Autodesk Inventor part; units mm, degrees
ref_plane "YZ Plane" through (0, 0, 0) normal (1, 0, 0) x (0, 1, 0)
ref_plane "XZ Plane" through (0, 0, 0) normal (0, 1, 0) x (-1, 0, 0)
ref_plane "XY Plane" through (0, 0, 0) normal (0, 0, 1) x (1, 0, 0)
sketch "Sketch1" plane through (0, 0, 0) normal (0, 1, 0) x (-1, 0, 0)
  circle A0 centre (0, 0) radius 6.35 construction
  line L0 (6.35, -3.6662) -> (0, -7.3323)
  line L1 (0, -7.3323) -> (-6.35, -3.6662)
  line L2 (-6.35, -3.6662) -> (-6.35, 3.6662)
  line L3 (-6.35, 3.6662) -> (0, 7.3323)
  line L4 (0, 7.3323) -> (6.35, 3.6662)
  line L5 (6.35, 3.6662) -> (6.35, -3.6662)
  circle A1 centre (0, 0) radius 9.525
  point P0 (6.35, 0)
  dimension "d0" = 12.7
  dimension "d1" = 19.05
extrude "Extrusion1" add sketch "Sketch1" along normal blind 9.525
properties part number "SportGearbox_HexDiffGearSpacer"
Geometry: final body of the model. Coordinates: model frame, mm. A direction names the side the tool comes from. Give positions to 0.01 mm unless a question says otherwise; leave off trailing zeros. Write each loop counter-clockwise with the first axis right and the second up, starting at its lowest first coordinate (ties: lowest second). Pieces come first, ordered by that corner, then holes.
1. Line query: probe 1 along X at (y, z) = (6.75, -2.25); probe 2 along X at (y, z) = (3.75, -0.25); probe 3 along Z at (x, y) = (1, 0.75). Output: solid intervals per line, ascending.
2. Section query B-B, the plane y = 5. Return loops of the section in (x, z) (3 decimals).
3. Section query A-A, the plane z = 0. Return loops of the section in (x, y) (3 decimals), then the cut area to 3 significant figures.
4. Section query C-C, the plane x = -3.5. Return loops of the section in (y, z) (3 decimals), then the cut area to 3 significant figures.
5. Pin query (flat end, axial travel): P1, Ø1, axis at x = -1.5, y = 8.5, coming from the -Z side; P2, Ø3, axis at y = 5.5, z = -4.5, coming from the +X side; P3, Ø2, axis at y = 7.5, z = 5.5, coming from the -X side (3 decimals). Return the tip coordinate at first contact, or that it passes through.
6. Draft query along Z for faces 3 (the flat face through (3.219, 4.696, 5.474)), 4 (the flat face through (6.35, 5, 0)), 5 (the cylindrical face through (7.559, 4.696, 5.796)), 6 (the flat face through (2.3, 0, -6.2)). Return one class per face: released by +Z, released by -Z, zero draft, split by the parting line, or undercut.
7. Reachability of faces 1 (the flat face through (-6.35, 5, 0)), 2 (the flat face through (2.3, 9.525, -6.2)) from +Z, -Z, +X, -X, +Y, -Y: full face, straight path, thin tool, end or side. Return the list, or none.
Computed:
1. probe 1: x = -9.26 to -6.35, 6.35 to 9.26
1. probe 2: x = -9.52 to -6.35, 6.35 to 9.52
1. probe 3: z = -9.47 to -6.75, 6.75 to 9.47
2. outline: circle Ø19.05 at (0, 0); hole (-6.35, -3.666) - (0, -7.332) - (6.35, -3.666) - (6.35, 3.666) - (0, 7.332) - (-6.35, 3.666) - close
3. outline: (-9.525, 0) - (-6.35, 0) - (-6.35, 9.525) - (-9.525, 9.525) - close; (6.35, 0) - (9.525, 0) - (9.525, 9.525) - (6.35, 9.525) - close
3. area: 60.5 mm2
4. outline: (0, -8.859) - (9.525, -8.859) - (9.525, -5.312) - (0, -5.312) - close; (0, 5.312) - (9.525, 5.312) - (9.525, 8.859) - (0, 8.859) - close
4. area: 67.6 mm2
5. P1: stops at z = -9.47
5. P2: stops at x = 9.04
5. P3: stops at x = -8.395
6. face 3: undercut
6. face 4: undercut
6. face 5: split by the parting line
6. face 6: zero draft
7. face 1: +Y, -Y
7. face 2: +Z, -Z, +X, -X, +Y
